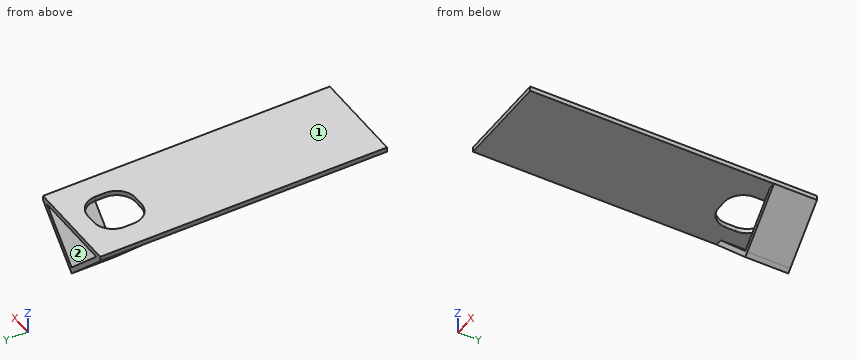
Autodesk Inventor part; units mm, degrees
ref_plane "YZ Plane" through (0, 0, 0) normal (1, 0, 0) x (0, 1, 0)
ref_plane "XZ Plane" through (0, 0, 0) normal (0, 1, 0) x (-1, 0, 0)
ref_plane "XY Plane" through (0, 0, 0) normal (0, 0, 1) x (1, 0, 0)
sketch "Sketch1" plane through (0, 0, 0) normal (0, 0, 1) x (1, 0, 0)
  line L0 (-50, -150) -> (50, -150)
  line L1 (50, -150) -> (50, 150)
  line L2 (50, 150) -> (-50, 150)
  line L3 (-50, 150) -> (-50, -150)
  line L4 (-50, -150) -> (50, 150) construction
  line L5 (50, -150) -> (-50, 150) construction
  point P0 (0, 0)
  dimension "d0" = 100
  dimension "d1" = 300
extrude "Extrusion1" add sketch "Sketch1" along normal blind 5
sketch "Sketch2" plane through (-50, 150, 0) normal (0, 1, 0) x (1, 0, 0)
  line L0 (0, 0) -> (100, 0)
  line L1 (0, 0) -> (49.9986, 49.9986)
  line L2 (49.9986, 49.9986) -> (53.5341, 46.463)
  line L3 (53.5341, 46.463) -> (3.5355, -3.5355)
  line L4 (3.5355, -3.5355) -> (0, 0)
  line L5 (0, 0) -> (70.7086, 0) construction
  line L6 (100.108, -0.1109) -> (53.5341, 46.463)
  line L7 (53.5341, 46.463) -> (49.9986, 42.9275)
  line L8 (49.9986, 42.9275) -> (96.5724, -3.6464)
  line L9 (96.5724, -3.6464) -> (100.108, -0.1109)
  point P0 (50, 0)
  point P1 (49.9986, 42.9275)
  dimension "d4" = 45
  dimension "d5" = 5
  dimension "d6" = 5
extrude "Extrusion2" add sketch "Sketch2" against normal blind 45 contours L1 L2 L3 L0 | L0 L3 L4 | L8 L3 L6 L0 | L0 L6 L9 L8
sketch "Sketch6" plane through (0, 0, 5) normal (0, 0, 1) x (1, 0, 0)
  line L0 (4.9986, 80) -> (-5.0014, 80)
  line L1 (-25.0014, 100) -> (-25.0014, 110)
  line L2 (-5.0014, 130) -> (4.9986, 130)
  line L3 (24.9986, 110) -> (24.9986, 100)
  line L4 (-0.0014, 150) -> (-0.0014, 105)
  line L5 (24.9986, 80) -> (-25.0014, 130) construction
  line L6 (-25.0014, 80) -> (24.9986, 130) construction
  arc A0 (4.9986, 80) -> (24.9986, 100) centre (4.9986, 100) ccw
  arc A1 (24.9986, 110) -> (4.9986, 130) centre (4.9986, 110) ccw
  arc A2 (-5.0014, 130) -> (-25.0014, 110) centre (-5.0014, 110) ccw
  arc A3 (-25.0014, 100) -> (-5.0014, 80) centre (-5.0014, 100) ccw
  point P0 (0, 0)
  dimension "d21" = 50
  dimension "d22" = 50
  dimension "d23" = 20
extrude "Extrusion6" cut sketch "Sketch6" against normal blind 5
properties part number "fixation_v05"
Model file for the job. Use its own axes, mm. Face numbers are marked on the shaded views. Coordinates: 2 decimals unless noted, no trailing zeros. Loops run counter-clockwise (first coordinate to the right, second up) from the corner with the lowest first, then second, coordinate; pieces in that order, holes last. Notation, with made-up numbers: (16, 34) - (42, 34) arc R12 cw to (42, 56) - close; hole circle Ø8 at (14, 83.25). An arc over 180 degrees is marked (long way). Answer as a JSON object with one key per item and string values. Group by question number.
(1) Two-plate mould, pull along X, no slides. Class the marked faces 1 and 2: released by +X, released by -X, zero draft, split by the parting line, or undercut.
(2) Flat gauge pins, fed straight in: pin 1 (1.5 mm diameter, centred on y = 73, z = 3, fed in from +X); pin 2 (1.5 mm diameter, centred on x = 7.5, z = -40.5, fed in from -Y). Where does each tip first touch, or does it go through?
(3) Cut at C-C (z = -11). Give the cut face in (x, y).
(4) Cut at D-D (x = -17). Give the cut face in (y, z), then the cut area to 3 significant figures.
(5) Cut at B-B (x = 11.5). Give the cut face in (y, z), then the cut area to 3 significant figures.
(6) Probe line 1 along Z through (x, y) = (-11.5, -62); line 2 along Y through (x, z) = (-6, -39.5); line 3 along X through (y, z) = (98, 1). List the from-to ranges inside material, lowest first.
(7) Cut at A-A (y = 93.5). Give the cut face in (x, z).
Geometry says:
{
 "1": {"face 1": "zero draft", "face 2": "undercut"},
 "2": {"pin 1": "stops at x = 50", "pin 2": "stops at y = 105"},
 "3": {"outline": "(-39, 105) - (-31.93, 105) - (-31.93, 150) - (-39, 150) - close; (31.93, 105) - (39, 105) - (39, 150) - (31.93, 150) - close"},
 "4": {"outline": "(-150, 0) - (84, 0) - (84, 5) - (-150, 5) - close; (105, -33) - (150, -33) - (150, -25.93) - (105, -25.93) - close; (126, 0) - (150, 0) - (150, 5) - (126, 5) - close", "area": "1,610 mm^2"},
 "5": {"outline": "(-150, 0) - (81.09, 0) - (81.09, 5) - (-150, 5) - close; (105, -38.5) - (150, -38.5) - (150, -31.43) - (105, -31.43) - close; (128.91, 0) - (150, 0) - (150, 5) - (128.91, 5) - close", "area": "1,580 mm^2"},
 "6": {"line 1": "z = 0 to 5", "line 2": "y = 105 to 150", "line 3": "x = -50 to -24.9, 24.9 to 50"},
 "7": {"outline": "(-50, 0) - (-23.92, 0) - (-23.92, 5) - (-50, 5) - close; (23.91, 0) - (50, 0) - (50, 5) - (23.91, 5) - close"}
}
